Autodesk Inventor part; units mm, degrees
ref_plane "YZ Plane" through (0, 0, 0) normal (1, 0, 0) x (0, 1, 0)
ref_plane "XZ Plane" through (0, 0, 0) normal (0, 1, 0) x (-1, 0, 0)
ref_plane "XY Plane" through (0, 0, 0) normal (0, 0, 1) x (1, 0, 0)
sketch "스케치1" plane through (0, 0, 0) normal (1, 0, 0) x (0, 1, 0)
  line L0 (46, 13.5) -> (0, 13.5)
  line L1 (0, 13.5) -> (0, -13.5)
  line L2 (0, -13.5) -> (46, -13.5)
  line L3 (46, -13.5) -> (46, 13.5)
  line L4 (39.5, 13.5) -> (39.5, 7.7432)
  line L5 (39.5, 5) -> (19, 5)
  line L6 (12.5, 5) -> (12.5, -5)
  line L7 (19, -5) -> (39.5, -5)
  line L8 (46, -5) -> (46, 5)
  line L9 (12.5, 5) -> (12.5, 13.5)
  line L10 (12.5, -5) -> (12.5, -13.5)
  line L11 (19, 13.5) -> (19, 5)
  line L12 (19, -5) -> (19, -13.5)
  line L13 (39.5, 5) -> (39.5, 7.7432)
  line L14 (39.5, -13.5) -> (39.5, -5)
  point P0 (0, 0)
  dimension "d0" = 27
  dimension "d1" = 13.5
  dimension "d2" = 46
  dimension "d3" = 10
  dimension "d4" = 5
  dimension "d5" = 12.5
  dimension "d7" = 39.5
  dimension "d8" = 39.5
revolve "회전1" add sketch "스케치1" angle 360 about axis through (0, 0, 13.5) along (0, 0, -1) contours L3 L2 L14 L7 L12 L10 L6 L9 L0 L11 L5 L13 L4
sketch "스케치2" plane through (0, 0, 13.5) normal (0, 0, 1) x (1, 0, 0)
  circle A0 centre (0, 0) radius 13
  dimension "d10" = 26
extrude "돌출1" cut sketch "스케치2" against normal blind 1
sketch "스케치3" plane through (0, 0, -13.5) normal (0, 0, -1) x (-1, 0, 0)
  circle A0 centre (0, 0) radius 13
  dimension "d13" = 26
extrude "돌출2" cut sketch "스케치3" against normal blind 1
fillet "모깎기1" radius 3 4 edges at (0, -46, 13.5) (0, -46, -13.5) (0, -19, 5) (0, -19, -5)
properties part number "2"
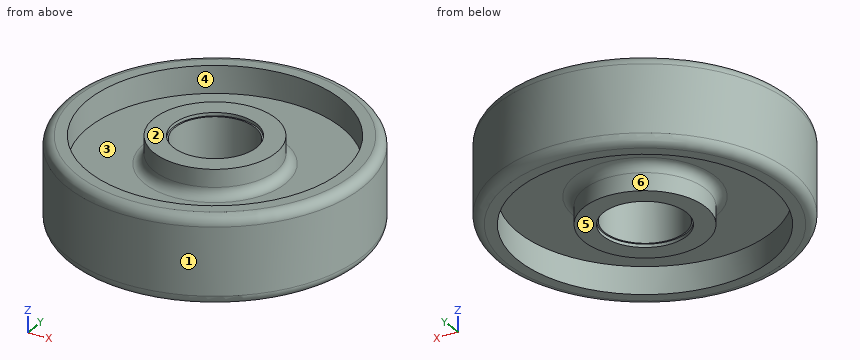
The listing builds one solid part. Answer for the finished solid, in the listing's coordinates (mm). Face numbers are marked on the shaded views. A direction names the side the tool comes from. Coordinates: 2 decimals unless noted, no trailing zeros. Loops run counter-clockwise (first coordinate to the right, second up) from the corner with the lowest first, then second, coordinate; pieces in that order, holes last. Notation, with made-up numbers: (30, 73) - (35, 73) arc R10 cw to (35, 82) - close; hole circle Ø7 at (75.25, 17). An arc over 180 degrees is marked (long way). Use a Markdown table: item, result. Add a question column.
1) The part is cut by section A-A, the plane z = 2.75. Give the vertices of the cut face in (x, y), and give its area (3 significant figures).
2) Given pin 1 (10 mm diameter, centred on x = 0, y = 28, fed in from -Z); pin 2 (10 mm diameter, centred on y = 16.5, z = 9, fed in from +X); pin 3 (5 mm diameter, centred on y = 10.5, z = -5, fed in from +X), each flat-ended and moving along its own axis, determine where each tip first touches the part or whether it passes through.
3) The part is cut by section B-B, the plane z = -6.5. Give the vertices of the cut face in (x, y).
4) For the marked faces 4, 5 and 6, determine the directions among +Z, -Z, +X, -X, +Y, -Y from which every point of the face is accessible in a straight line to the end or side of a thin tool.
5) Find the intervals of material crossed by line 1 (X direction, y = 0, z = 8.75); line 2 (Y direction, x = -13, z = -5.5); line 3 (X direction, y = -1, z = 11.25), in increasing order.
6) The mould has two halves that part along Y. Classify the marked faces 1, 2 and 3: released by +Y, released by -Y, zero draft, split by the parting line, or undercut.
Here are the results:
| question | item | result |
|---|---|---|
| 1 | outline | circle Ø92 at (0, 0); hole circle Ø25 at (0, 0) |
| 1 | area | 6,160 mm^2 |
| 2 | pin 1 | stops at z = -5 |
| 2 | pin 2 | stops at x = 44.54 |
| 2 | pin 3 | stops at x = 45.3 |
| 3 | outline | circle Ø92 at (0, 0); circle Ø38.8 at (0, 0); hole circle Ø79 at (0, 0); hole circle Ø25 at (0, 0) |
| 4 | face 4 | +Z |
| 4 | face 5 | -Z, +X, -X, +Y, -Y |
| 4 | face 6 | -Z |
| 5 | line 1 | x = -46 to -39.5, -19 to -12.5, 12.5 to 19, 39.5 to 46 |
| 5 | line 2 | y = -44.12 to -37.3, -15.65 to 15.65, 37.3 to 44.12 |
| 5 | line 3 | x = -45.89 to -39.49, -18.97 to -12.46, 12.46 to 18.97, 39.49 to 45.89 |
| 6 | face 1 | split by the parting line |
| 6 | face 2 | zero draft |
| 6 | face 3 | undercut |
